The listing builds one solid part. Answer for the finished solid, in the listing's coordinates (mm). A direction names the side the tool comes from. Give positions to 0.01 mm unless a question says otherwise; leave off trailing zeros. Order: outer loops, then holes, each group sorted by start corner. A loop starts at its lowest first (then second) coordinate and runs counter-clockwise, first axis right, second up. Notation, with made-up numbers: (-33.75, 40.5) - (-26.75, 40.5) arc R28 cw to (-26.75, 62.5) - close; hole circle Ø6 at (22, 37.5). An arc over 180 degrees is marked (long way). Use CSV: the item, a comma, the result in double quotes.
```python
from build123d import *

# Parameters (mm, degrees)
F1_DEPTH = 63.5
F0_W     = 25.4
F0_H     = 19.05
F2_DEPTH = 25.4
F3_DEPTH = 7.9375


with BuildPart() as f1:
    # F0 (on Front) → F1 (new body, symmetric)
    with BuildSketch(Plane.XZ):
        Polygon((22.225, 9.525), (-41.275, 9.525), (-41.275, -9.525), (41.275, -9.525), (41.275, 9.525), align=None)
    extrude(amount=F1_DEPTH, both=True)

    # F0 (on Front) → F2 (join, symmetric)
    with BuildSketch(Plane.XZ):
        with BuildLine():
            Line((22.225, 27.0002), (22.225, 9.525))
            Line((22.225, 9.525), (41.275, 9.525))
            Line((41.275, 9.525), (41.275, 27.0002))
            ThreePointArc((41.275, 27.0002), (45.9246798487, 38.2255201513), (57.15, 42.8752))
            Line((57.15, 42.8752), (85.725, 42.8752))
            Line((85.725, 42.8752), (85.725, 61.9252))
            Line((85.725, 61.9252), (57.15, 61.9252))
            ThreePointArc((57.15, 61.9252), (32.4542956671, 51.6959043329), (22.225, 27.0002))
        make_face()
        with Locations((98.425, 52.4002)):
            Rectangle(F0_W, F0_H)
    extrude(amount=F2_DEPTH, both=True)

    # F0 (on Front) → F3 (join, symmetric)
    with BuildSketch(Plane.XZ):
        with BuildLine():
            add(Edge.make_bspline(
                [(-41.275, 9.525), (-41.2765443325, 43.204266578), (5.9362053871, 72.3337382078), (57.15, 61.9252)],
                knots=[0, 0, 0, 0, 111.5045361635, 111.5045361635, 111.5045361635, 111.5045361635], degree=3))
            Line((-41.275, 9.525), (22.225, 9.525))
            Line((22.225, 9.525), (22.225, 27.0002))
            ThreePointArc((22.225, 27.0002), (32.4542956671, 51.6959043329), (57.15, 61.9252))
        make_face()
    extrude(amount=F3_DEPTH, both=True)

    # F0 (on Front) → F4 (revolve)
    with BuildSketch(Plane.XZ):
        Polygon((111.125, 66.675), (111.125, 61.9252), (111.125, 42.8752), (111.125, 38.1), (136.525, 38.1), (136.525, 66.675), align=None)
    revolve(axis=Axis((111.125, 0, 52.3875), (0, 0, -1)))


with BuildPart() as f5_1:
    # F5: copy of F1
    add(f1.part)


with BuildPart() as f6_1:
    # F6: copy of F1
    add(f1.part.moved(Location((50.8, 50.8, 50.8))))


solid = f1.part
```
Item 1: Which of the six approach directions +Z, -Z, +X, -X, +Y, -Y give full straight-line access (tool end or side, diameter ignored) to faces 4 (the face through (56, 25.4, 48)), 5 (the face through (56, -25.4, 48)), 6 (the face through (45.8, -0.4, 38.1)), 7 (the face through (22.225, 17, 18)), 8 (the face through (41.275, -1, 4))?
Taken from the geometry:
face 4,"+Z, +X, -X, +Y"
face 5,"+Z, +X, -X, -Y"
face 6,"-Z, +Y, -Y"
face 7,"+Z, -X, +Y"
face 8,"-Z, +X, +Y, -Y"
Item 2: The part is cut by section A-A (y = 20). Give the vertices of the cut face in (x, z) (3 decimals).
Taken from the geometry:
outline,"(-41.275, -9.525) - (41.275, -9.525) - (41.275, 27) arc R15.875 cw to (57.15, 42.875) - (95.467, 42.875) - (95.467, 38.1) - (126.783, 38.1) - (126.783, 66.675) - (95.467, 66.675) - (95.467, 61.925) - (57.15, 61.925) arc R34.925 ccw to (22.225, 27) - (22.225, 9.525) - (-41.275, 9.525) - close"
Item 3: Each of these flat-tipped pins is pushed along its axis until it touches: pin 1 (3 mm diameter, centred on y = -12, z = 24, fed in from -X) (3 decimals); pin 2 (2 mm diameter, centred on x = 9, z = 35.5, fed in from -Y); pin 3 (16.5 mm diameter, centred on x = -17.5, y = -23, fed in from +Z) (3 decimals); pin 4 (19 mm diameter, centred on y = -20.5, z = 14.5, fed in from -X) (3 decimals). Where does it stop, or does it pass through?
Taken from the geometry:
pin 1,"x = 22.225"
pin 2,"y = -7.94"
pin 3,"z = 9.525"
pin 4,"x = -41.275"
Item 4: Find the intervals of material crossed by line 1 along Z through (x, y) = (101.5, 3) (3 decimals); line 2 along Z through (x, y) = (-30.5, -38) (3 decimals); line 3 along X through (y, z) = (2, -3) (3 decimals), in increasing order.
Taken from the geometry:
line 1,"38.1 to 66.675"
line 2,"-9.525 to 9.525"
line 3,"-41.275 to 41.275"
Item 5: The part is cut by section C-C (y = -49). Give the vertices of the cut face in (x, z) (3 decimals), and give its area (3 significant figures).
Taken from the geometry:
outline,"(-41.275, -9.525) - (41.275, -9.525) - (41.275, 9.525) - (-41.275, 9.525) - close"
area,"1,570 mm^2"
Item 6: The mould has two halves that part along X. Classify faces 1 (the face through (32.73, -16.79, 51.97)), 2 (the face through (-2, -7.938, 34)), 3 (the face through (72, 0, 42.875)): +X half, -X half, draft (parallel to the pull), parting line (faces both ways), or undercut.
Taken from the geometry:
face 1,"-X half"
face 2,"draft"
face 3,"undercut"
Item 7: The part is cut by section B-B (x = 71.5). Give the vertices of the cut face in (y, z), and give its area (3 significant figures).
Taken from the geometry:
outline,"(-25.4, 42.88) - (25.4, 42.88) - (25.4, 61.93) - (-25.4, 61.93) - close"
area,"968 mm^2"
